Build history of the part. All positions in model axes, mm. A direction names the side the tool comes from. Round coordinates to 2 decimals unless told otherwise and drop trailing zeros. Order: outer loops, then holes, each group sorted by start corner. A loop starts at its lowest first (then second) coordinate and runs counter-clockwise, first axis right, second up. Notation, with made-up numbers: (74, 56) -> (123, 56) arc R23 cw to (123, 71) -> close; hole circle Ø1 at (-23, 37). An arc over 180 degrees is marked (long way). Use a Markdown table: item, result. Add a question column.
Item 1: Slice it at A-A, the plane z = -13. Give the cut face in (x, y), plus the area to 3 significant figures.
Item 2: Slice it at C-C, the plane y = -2.75. Give the cut face in (x, z).
Item 3: Slice it at D-D, the plane x = 11. Give the cut face in (y, z), plus the area to 3 significant figures.
Item 4: 3-axis set-ups, long thin cutter, end or side, ignore diameter. For faces 1 (the face through (12, -5, -25)), 2 (the face through (16, 19, -25)), 3 (the face through (12, 14, -25)): which of +Z, -Z, +X, -X, +Y, -Y reach the whole face in a straight line?
Item 5: Slice it at B-B, the plane x = 15.5. Give the cut face in (y, z).
Item 6: Pin check, flat tips, straight feed: pin 1 (3.5 mm diameter, centred on x = 8, z = -23, fed in from -Y); pin 2 (12 mm diameter, centred on y = 11.5, z = -31.5, fed in from -X); pin 3 (6 mm diameter, centred on x = 6, y = -0.5, fed in from +Z); pin 4 (4 mm diameter, centred on y = -6.24, z = -15.32, fed in from -X). Stop position of each tip, or through.
Item 7: Probe L1, parallel to Y at x = 2.5, z = -14; L2, parallel to X at y = 11.25, z = -29; L3, parallel to Z at x = 13.75, y = -6.5. List the from-to ranges inside material, lowest first.
from build123d import *

# Parameters (mm, degrees)
SKETCH1_W           = 20
SKETCH1_H           = 50
BOSS_EXTRUDE1_DEPTH = 8
FILLET1_R           = 10
SKETCH2_W           = 50
SKETCH2_H           = 30
BOSS_EXTRUDE2_DEPTH = 8
SKETCH3_R           = 1.5
CUT_EXTRUDE1_DEPTH  = 8


with BuildPart() as part:
    # Sketch1 → Boss-Extrude1 (new body)
    with BuildSketch(Plane(origin=(0, 0, 0), x_dir=(1, 0, 0), z_dir=(0, 1, 0))):
        with Locations((10, 25)):
            Rectangle(SKETCH1_W, SKETCH1_H)
    extrude(amount=BOSS_EXTRUDE1_DEPTH)

    # Fillet1
    fillet1_edges = [part.edges().sort_by_distance(p)[0] for p in [
        (0, 4, -50),
        (0, 4, 0),
    ]]
    fillet(fillet1_edges, radius=FILLET1_R)

    # Sketch2 → Boss-Extrude2 (add)
    with BuildSketch(Plane(origin=(20, 0, 0), x_dir=(0, 0, -1), z_dir=(1, 0, 0))):
        with Locations((25, 4)):
            Rectangle(SKETCH2_W, SKETCH2_H)
    extrude(amount=-BOSS_EXTRUDE2_DEPTH)

    # Sketch3 → Cut-Extrude1 (cut)
    with BuildSketch(Plane(origin=(20, 0, 0), x_dir=(0, 0, -1), z_dir=(1, 0, 0))):
        with Locations((15.311973507, 13.760568851)):
            Circle(SKETCH3_R)
        with Locations((15.324315829, -6.23942734)):
            Circle(SKETCH3_R)
        with Locations((35.311973507, 13.760568851)):
            Circle(SKETCH3_R)
        with Locations((35.324315829, -6.23942734)):
            Circle(SKETCH3_R)
    extrude(amount=-CUT_EXTRUDE1_DEPTH, mode=Mode.SUBTRACT)


solid = part.part
Check sheet entries:
| question | item | result |
|---|---|---|
| 1 | outline | (0, 0) -> (12, 0) -> (12, -11) -> (20, -11) -> (20, 19) -> (12, 19) -> (12, 8) -> (0, 8) -> close |
| 1 | area | 336 mm2 |
| 2 | outline | (12, -50) -> (20, -50) -> (20, 0) -> (12, 0) -> close |
| 3 | outline | (0, -50) -> (8, -50) -> (8, 0) -> (0, 0) -> close |
| 3 | area | 400 mm2 |
| 4 | face 1 | +Z, -Z, -X, -Y |
| 4 | face 2 | +Z, -Z, +X, -X, +Y |
| 4 | face 3 | +Z, -Z, -X, +Y |
| 5 | outline | (-11, -50) -> (19, -50) -> (19, 0) -> (-11, 0) -> close; hole circle Ø3 at (-6.24, -35.32); hole circle Ø3 at (-6.24, -15.32); hole circle Ø3 at (13.76, -35.31); hole circle Ø3 at (13.76, -15.31) |
| 6 | pin 1 | y = 0 |
| 6 | pin 2 | x = 0 |
| 6 | pin 3 | z = -0.05 |
| 6 | pin 4 | x = 12 |
| 7 | L1 | 0 to 8 |
| 7 | L2 | 12 to 20 |
| 7 | L3 | -50 to -36.8, -33.85 to -16.8, -13.85 to 0 |
